Study the drawing (mm; zero at the part's minimum x, y, z) and answer. A direction names the side the tool comes from. Give positions to 0.01 mm unless a question says otherwise; leave off trailing zeros. Order: outer loops, then holes, each group sorted by start corner. A loop starts at its lowest first (then second) coordinate and runs counter-clockwise, first axis right, second up. Notation, with made-up numbers: (32, -5) - (81, -5) arc R26 cw to (81, 16) - close; hole circle Ø2 at (18, 0.5). An arc over 180 degrees is marked (long way). Put each result on its own line as item: value.
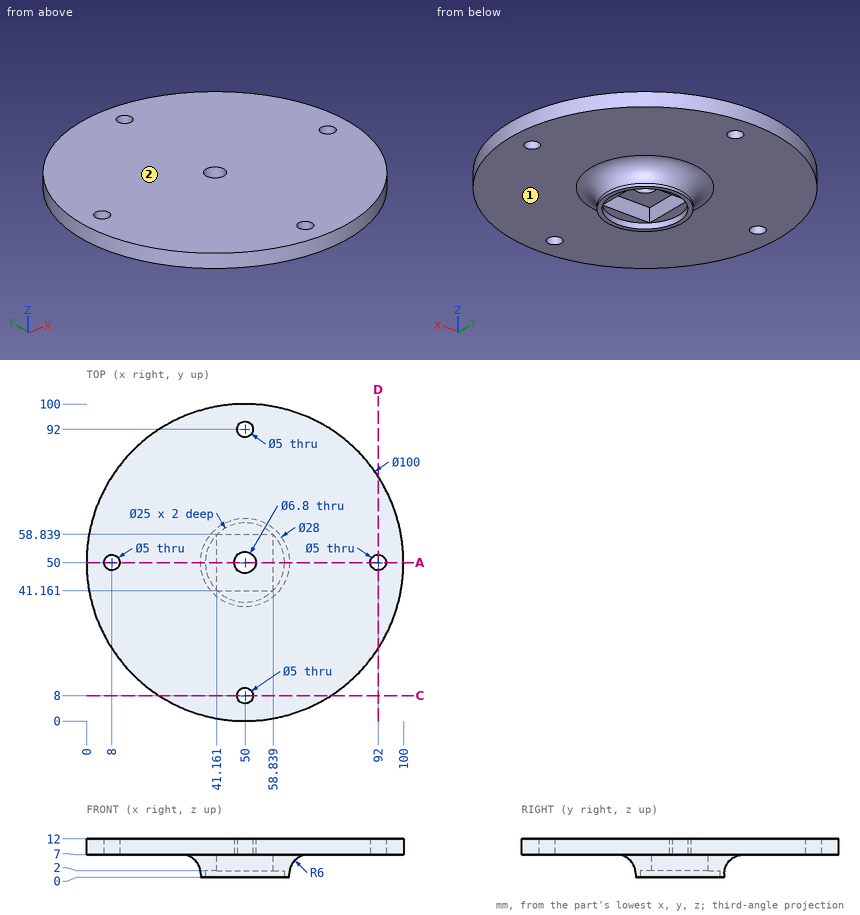
(1) Straight lines are drawn through the part: line 1 (Y direction, x = 50, z = 8.95); line 2 (Y direction, x = 50, z = 0.5); line 3 (Z direction, x = 58.5, y = 48). For each, find the intervals that lie inside material, in ascending order.
Geometry check:
line 1: y = 0 to 5.5, 10.5 to 46.6, 53.4 to 89.5, 94.5 to 100
line 2: y = 36 to 37.5, 62.5 to 64
line 3: z = 7 to 12
(2) Section A-A, the plane y = 50 is taken. Count the separate pieces of the cut face and the enclosed holes in it, then the cut area to 3 significant figures.
Geometry check:
separate pieces: 4
enclosed holes: 0
area: 489 mm²
(3) Given pin 1 (8 mm diameter, centred on x = 50, y = 50, fed in from -Z); pin 2 (1.1 mm diameter, centred on x = 60.5, y = 54, fed in from -Z); pin 3 (2 mm diameter, centred on y = 23.5, z = 10, fed in from -X), each flat-ended and moving along its own axis, determine where each tip first touches the part or whether it passes through.
Geometry check:
pin 1: stops at z = 7
pin 2: stops at z = 2
pin 3: stops at x = 6.99
(4) A tool of negligible diameter and unlimited length cuts with its end or side. For the marked faces 1 and 2, from which of +Z, -Z, +X, -X, +Y, -Y can it reach the whole face along a straight path? Write none if from no direction.
Geometry check:
face 1: -Z
face 2: +Z, +X, -X, +Y, -Y
(5) Section C-C, the plane y = 8 is taken. Write down the section's boundary in (x, z).
Geometry check:
outline: (22.87, 7) - (47.5, 7) - (47.5, 12) - (22.87, 12) - close; (52.5, 7) - (77.13, 7) - (77.13, 12) - (52.5, 12) - close
